The model under review builds one solid part; all positions refer to its coordinate system, in mm. A direction names the side the tool comes from. Coordinates: 2 decimals unless noted, no trailing zeros. Order: outer loops, then holes, each group sorted by start corner. A loop starts at its lowest first (then second) coordinate and runs counter-clockwise, first axis right, second up. Notation, with made-up numbers: M 20.25,38.5 L 32.25,38.5 A18 cw 32.25,72.5 Z; hole C 49,-14 d7. An arc over 180 degrees is marked long. One line per item, written item: value.
```python
from build123d import *

# Parameters (mm, degrees)
SKETCH1_W           = 30
SKETCH1_H           = 30
BOSS_EXTRUDE1_DEPTH = 10
SKETCH2_W           = 20
SKETCH2_H           = 20
BOSS_EXTRUDE2_DEPTH = 20
CUT_EXTRUDE3_DEPTH  = 10


with BuildPart() as part:
    # Sketch1 → Boss-Extrude1 (new body)
    with BuildSketch(Plane(origin=(0, 0, 0), x_dir=(1, 0, 0), z_dir=(0, 1, 0))):
        Rectangle(SKETCH1_W, SKETCH1_H)
    extrude(amount=BOSS_EXTRUDE1_DEPTH)

    # Sketch2 → Boss-Extrude2 (add)
    with BuildSketch(Plane(origin=(-19.996706831, 6.023656636, 0.235617172), x_dir=(-0.9916527006816696, -0.12883913939699687, -0.005039582343056198), z_dir=(0.12893766412786933, -0.9908949522292337, -0.03875915912237427))):
        with Locations((-20.018899737, -0.342067519)):
            Rectangle(SKETCH2_W, SKETCH2_H)
    extrude(amount=-BOSS_EXTRUDE2_DEPTH)

    # Sketch5 → Cut-Extrude3 (cut)
    with BuildSketch(Plane(origin=(-2.292112058, 28.477077557, 1.107866318), x_dir=(0.9916435574745326, 0.12900579254219657, 0.0007486052452988832), z_dir=(-0.12893766412786928, 0.9908949522292337, 0.03875915912237423))):
        Polygon((-3.672779426, -10.332409771), (-3.672779426, -3.610260169), (-10.450784263, -3.610260169), (-10.479525344, -10.303179891), align=None)
        Polygon((2.827220574, -10.360322406), (2.827220574, -3.610200238), (9.549400399, -3.610200238), (9.520290252, -10.389064131), align=None)
        Polygon((-10.393641105, 9.696635705), (-3.672779426, 9.667774634), (-3.672779426, 2.889739831), (-10.422871628, 2.889739831), align=None)
        Polygon((9.606174491, 9.610751466), (9.577312777, 2.889739831), (2.827220574, 2.889739831), (2.827220574, 9.639861999), align=None)
    extrude(amount=-CUT_EXTRUDE3_DEPTH, mode=Mode.SUBTRACT)


solid = part.part
```
(1) For L1, parallel to Y at x = -13.5, z = -3; L2, parallel to Y at x = -1, z = -4.5; L3, parallel to X at y = 13, z = 6, list the stretches that pass through material, from the lowest coordinate up.
Geometry results:
L1: y = 0 to 10
L2: y = 0 to 28.86
L3: x = -10.83 to 9.34
(2) We need section A-A, the plane x = -6.5. State the section outline as (y, z) points.
Geometry results:
outline: M 0,-15 L 10,-15 L 10,-9.27 L 18.23,-8.95 L 17.97,-2.17 L 28.04,-1.78 L 27.79,4.71 L 17.71,4.32 L 17.45,11.03 L 10,10.74 L 10,15 L 0,15 Z
(3) Mouldability with a two-part tool opening along X and no side actions: class faces 4 (the flat face through (5.18, 19.62, -5.58)), 5 (the flat face through (-2.58, 28.43, 1.31)), 6 (the flat face through (0, 0, 0)) as +X half, -X half, draft (parallel to the pull), parting line (faces both ways), or undercut.
Geometry results:
face 4: undercut
face 5: -X half
face 6: draft
(4) We need section D-D, the plane z = -0.5. State the section outline as (x, y) points, plus the area to 3 significant figures.
Geometry results:
outline: M -15,0 L 15,0 L 15,10 L 9.76,10 L 7.19,29.77 L -12.64,27.19 L -10.41,10 L -15,10 Z
area: 673 mm2
(5) We need section C-C, the plane z = -7.75. State the section outline as (x, y) points.
Geometry results:
outline: M -15,0 L 15,0 L 15,10 L 8.16,10 L 9.77,10.21 L 8.48,20.13 L 1.76,19.26 L 0.47,29.18 L -5.97,28.34 L -4.68,18.42 L -11.35,17.55 L -10.37,10 L -15,10 Z
(6) Tool access review of faces 1 (the flat face through (-8.038, 17.382, 7.634)), 2 (the flat face through (-1.03, 16.1, 10.98)), 3 (the flat face through (-7.97, 17.91, -5.62)): name each direction out of +Z, -Z, +X, -X, +Y, -Y from which nothing blocks a thin tool from reaching the whole face with its end or side.
Geometry results:
face 1: +Z, -X
face 2: +Z, +X, -X
face 3: -X
(7) We need section B-B, the plane y = 21.25. State the section outline as (x, z) points, plus the area to 3 significant figures.
Geometry results:
outline: M -11.89,4.48 L -11.86,-2.02 L -5.05,-2.05 L -5.05,-8.83 L 1.51,-8.83 L 1.5,-2.08 L 8.31,-2.11 L 8.28,4.4 L 1.5,4.43 L 1.49,11.18 L -5.06,11.18 L -5.06,4.45 Z
area: 220 mm2
(8) Insertion check: pin 1 Ø1 at (x, y) = (-8.5, 19.5) entering from +Z; pin 2 Ø15 at (x, z) = (-4, -0.5) entering from +Y; pin 3 Ø6 at (x, y) = (-6.5, 16) entering from +Z. Each pin has a flat end and moves straight along its axis. Give the tip position at first contact, or say it passes through.
Geometry results:
pin 1: stops at z = 4.42
pin 2: stops at y = 29.33
pin 3: stops at z = 11.07
